from build123d import *

# Parameters (mm, degrees)
SKETCH1_W           = 145
SKETCH1_H           = 40
SKETCH1_R           = 2.5
SKETCH1_R_2         = 3.3
BOSS_EXTRUDE1_DEPTH = 9
FILLET1_R           = 1


with BuildPart() as part:
    # Sketch1 → Boss-Extrude1 (new body)
    with BuildSketch(Plane(origin=(0, 0, 0), x_dir=(1, 0, 0), z_dir=(0, 1, 0))):
        Rectangle(SKETCH1_W, SKETCH1_H)
        with Locations(Location((26.5, 0, 0), (0, 0, 270))):
            Circle(SKETCH1_R, mode=Mode.SUBTRACT)
        with Locations(Location((62.5, -12.5, 0), (0, 0, 270))):
            Circle(SKETCH1_R_2, mode=Mode.SUBTRACT)
        with Locations(Location((62.5, 12.5, 0), (0, 0, 90))):
            Circle(SKETCH1_R_2, mode=Mode.SUBTRACT)
        with Locations(Location((-26.5, 0, 0), (0, 0, 90))):
            Circle(SKETCH1_R, mode=Mode.SUBTRACT)
        with Locations(Location((-62.5, 12.5, 0), (0, 0, 90))):
            Circle(SKETCH1_R_2, mode=Mode.SUBTRACT)
        with Locations(Location((-62.5, -12.5, 0), (0, 0, 270))):
            Circle(SKETCH1_R_2, mode=Mode.SUBTRACT)
    extrude(amount=BOSS_EXTRUDE1_DEPTH)

    # Fillet1
    fillet1_edges = [part.edges().sort_by_distance(p)[0] for p in [
        (72.5, 4.5, 20),
        (-72.5, 4.5, 20),
        (-72.5, 4.5, -20),
        (72.5, 4.5, -20),
    ]]
    fillet(fillet1_edges, radius=FILLET1_R)


solid = part.part
Could you check a few things on this model? Use its own coordinates, in mm. Give positions to 0.01 mm unless a question says otherwise; leave off trailing zeros. Order: outer loops, then holes, each group sorted by start corner. A loop starts at its lowest first (then second) coordinate and runs counter-clockwise, first axis right, second up.
Item 1: If we section it at A-A, the plane z = 12.5: Write out the boundary of the cut face in (x, y).
Item 2: If we section it at B-B, the plane x = 62.5: Write out the boundary of the cut face in (y, z).
Item 3: I need wall thicknesses on line 1 (X direction, y = 4.5, z = 0); line 2 (X direction, y = 3.25, z = 12.5); line 3 (Z direction, x = -26.5, y = 5). Which ranges of each line are inside material? Lowest first, please.
Item 4: If we section it at C-C, the plane y = 7: Write out the boundary of the cut face in (x, z).
Item 5: I'm going to push a flat-ended pin straight in: pin 1 (5.5 mm diameter, centred on x = 62.5, z = -12.5, fed in from -Y). Where does the tip first touch, or does it pass through?
Item 6: If we mould it in two halves opening along Z, with no side actions, what happens to faces 1 (the face through (-1, 9, 0)), 2 (the face through (-1, 4, 20)), 3 (the face through (65.77, 4.44, 12.07)), 4 (the face through (-1, 4, -20))? For each: pulls with the +Z half, pulls with the -Z half, needs draft (parallel to the pull), parting line crosses it, or undercut.
Item 7: If we section it at D-D, the plane x = -26.5: Write out the boundary of the cut face in (y, z), plus the area to 3 significant figures.
Values:
1. outline: (-72.5, 0) - (-65.8, 0) - (-65.8, 9) - (-72.5, 9) - close; (-59.2, 0) - (59.2, 0) - (59.2, 9) - (-59.2, 9) - close; (65.8, 0) - (72.5, 0) - (72.5, 9) - (65.8, 9) - close
2. outline: (0, -20) - (9, -20) - (9, -15.8) - (0, -15.8) - close; (0, -9.2) - (9, -9.2) - (9, 9.2) - (0, 9.2) - close; (0, 15.8) - (9, 15.8) - (9, 20) - (0, 20) - close
3. line 1: x = -72.5 to -29, -24 to 24, 29 to 72.5
3. line 2: x = -72.5 to -65.8, -59.2 to 59.2, 65.8 to 72.5
3. line 3: z = -20 to -2.5, 2.5 to 20
4. outline: (-72.5, -19) arc R1 ccw to (-71.5, -20) - (71.5, -20) arc R1 ccw to (72.5, -19) - (72.5, 19) arc R1 ccw to (71.5, 20) - (-71.5, 20) arc R1 ccw to (-72.5, 19) - close; hole circle Ø6.6 at (-62.5, -12.5); hole circle Ø6.6 at (-62.5, 12.5); hole circle Ø5 at (-26.5, 0); hole circle Ø5 at (26.5, 0); hole circle Ø6.6 at (62.5, -12.5); hole circle Ø6.6 at (62.5, 12.5)
5. pin 1: passes through
6. face 1: needs draft
6. face 2: pulls with the +Z half
6. face 3: undercut
6. face 4: pulls with the -Z half
7. outline: (0, -20) - (9, -20) - (9, -2.5) - (0, -2.5) - close; (0, 2.5) - (9, 2.5) - (9, 20) - (0, 20) - close
7. area: 315 mm2
